Here's how the part is built. I have some questions about the finished solid (model axes, mm). Face numbers are marked on the shaded views. A direction names the side the tool comes from. Coordinates: 2 decimals unless noted, no trailing zeros. Write each loop counter-clockwise with the first axis right and the second up, starting at its lowest first coordinate (ties: lowest second). Pieces come first, ordered by that corner, then holes.
Item 1: I'm going to push flat-ended pins straight in: pin 1 Ø4 at (y, z) = (0, 8) entering from +X; pin 2 Ø4 at (y, z) = (14.5, 8.5) entering from +X; pin 3 Ø2.5 at (y, z) = (18, 7) entering from -X; pin 4 Ø1 at (x, z) = (5.5, 6.5) entering from -Y. Where does each tip first touch, or does it pass through?
Item 2: If we section it at C-C (y = -4): Please give me the cut outline in (x, z), then the cut area to 3 significant figures.
Item 3: For the marked faces 5, 6 and 7, which set-ups out of +Z, -Z, +X, -X, +Y, -Y let a thin tool reach every point of the face, with its end or its side?
Item 4: If we section it at B-B (z = 6): Please give me the cut outline in (x, y), then the cut area to 3 significant figures.
Item 5: If we section it at D-D (z = 8.25): Count the separate pieces of the cut face and the enclosed holes in it, then the cut area to 3 significant figures.
Item 6: We'd pull the mould along Y, two halves only. Please class the marked faces 1, 2, 3 and 4: +Y half, -Y half, draft (parallel to the pull), parting line (faces both ways), or undercut.
Item 7: If we section it at A-A (x = 0): Please give me the cut outline in (y, z), then the cut area to 3 significant figures.
Item 8: If I drill on line 1 (Y direction, x = 0, z = 2.75); line 2 (X direction, y = -6.5, z = 10.75); line 3 (Y direction, x = 0, z = 5.25), over which ranges is the centre line in solid material (lowest first)?
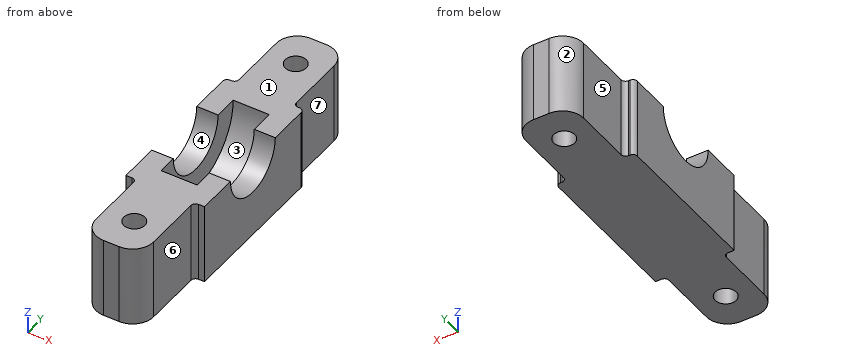
from build123d import *

# Parameters (mm, degrees)
F0_R     = 1.5
F0_W     = 5.1
F0_H     = 16.1
F1_DEPTH = 11.5
F3_DEPTH = 25


# Not quite as in the source:
# - a feature names something its author has since deleted; it is built from what else it names


with BuildPart() as f1:
    # F0 (on Top) → F1 (new body)
    with BuildSketch(Plane.XY):
        with BuildLine():
            ThreePointArc((5.5999997705, 10.465261464), (5.4140892248, 10.9140892248), (4.965261464, 11.0999997705))
            Line((4.965261464, 11.0999997705), (4.734738077, 11.0999997705))
            Line((4.734738077, 11.0999997705), (-4.734738077, 11.0999997705))
            Line((-4.734738077, 11.0999997705), (-4.965261464, 11.0999997705))
            ThreePointArc((-4.965261464, 11.0999997705), (-5.4140892248, 10.9140892248), (-5.5999997705, 10.465261464))
            Line((-5.5999997705, 10.465261464), (-5.5999997705, -10.465261464))
            ThreePointArc((-5.5999997705, -10.465261464), (-5.4140892248, -10.9140892248), (-4.965261464, -11.0999997705))
            Line((-4.965261464, -11.0999997705), (-4.734738077, -11.0999997705))
            Line((-4.734738077, -11.0999997705), (4.734738077, -11.0999997705))
            Line((4.734738077, -11.0999997705), (4.965261464, -11.0999997705))
            ThreePointArc((4.965261464, -11.0999997705), (5.4140892248, -10.9140892248), (5.5999997705, -10.465261464))
            Line((5.5999997705, -10.465261464), (5.5999997705, 10.465261464))
        make_face()
        Polygon((2.6, 8.1), (2.6, 0), (2.6, -8.1), (-2.6, -8.1), (-2.6, 8.1), align=None, mode=Mode.SUBTRACT)
        with BuildLine():
            Line((-4.734738077, 11.0999997705), (4.734738077, 11.0999997705))
            ThreePointArc((4.734738077, 11.0999997705), (4.2859103162, 11.2859103162), (4.0999997705, 11.734738077))
            Line((4.0999997705, 11.734738077), (4.0999997705, 20.0999997705))
            ThreePointArc((4.0999997705, 20.0999997705), (3.2213201141, 22.2213201141), (1.0999997705, 23.0999997705))
            Line((1.0999997705, 23.0999997705), (-1.0999997705, 23.0999997705))
            ThreePointArc((-1.0999997705, 23.0999997705), (-3.2213201141, 22.2213201141), (-4.0999997705, 20.0999997705))
            Line((-4.0999997705, 20.0999997705), (-4.0999997705, 11.734738077))
            ThreePointArc((-4.0999997705, 11.734738077), (-4.2859103162, 11.2859103162), (-4.734738077, 11.0999997705))
        make_face()
        with Locations((0, 18)):
            Circle(F0_R, mode=Mode.SUBTRACT)
        with BuildLine():
            ThreePointArc((4.0999997705, -11.734738077), (4.2859103162, -11.2859103162), (4.734738077, -11.0999997705))
            Line((4.734738077, -11.0999997705), (-4.734738077, -11.0999997705))
            ThreePointArc((-4.734738077, -11.0999997705), (-4.2859103162, -11.2859103162), (-4.0999997705, -11.734738077))
            Line((-4.0999997705, -11.734738077), (-4.0999997705, -20.0999997705))
            ThreePointArc((-4.0999997705, -20.0999997705), (-3.2213201141, -22.2213201141), (-1.0999997705, -23.0999997705))
            Line((-1.0999997705, -23.0999997705), (1.0999997705, -23.0999997705))
            ThreePointArc((1.0999997705, -23.0999997705), (3.2213201141, -22.2213201141), (4.0999997705, -20.0999997705))
            Line((4.0999997705, -20.0999997705), (4.0999997705, -11.734738077))
        make_face()
        with Locations((0, -18)):
            Circle(F0_R, mode=Mode.SUBTRACT)
        Polygon((2.6, -8.1), (2.6, 0), (2.6, 8.1), (-2.6, 8.1), (-2.6, -8.1), align=None)
        Rectangle(F0_W, F0_H, mode=Mode.SUBTRACT)
        Rectangle(F0_W, F0_H)
        with BuildLine():
            Line((5.5999997705, -11.0999997705), (5.5999997705, -10.465261464))
            ThreePointArc((5.5999997705, -10.465261464), (5.4140892248, -10.9140892248), (4.965261464, -11.0999997705))
            Line((4.965261464, -11.0999997705), (5.5999997705, -11.0999997705))
        make_face()
        with BuildLine():
            ThreePointArc((-4.965261464, -11.0999997705), (-5.4140892248, -10.9140892248), (-5.5999997705, -10.465261464))
            Line((-5.5999997705, -10.465261464), (-5.5999997705, -11.0999997705))
            Line((-5.5999997705, -11.0999997705), (-4.965261464, -11.0999997705))
        make_face()
    extrude(amount=F1_DEPTH)

    # F2 (on face) → F3 (cut)
    with BuildSketch(Plane.YZ.offset(5.5999997705)):
        with BuildLine():
            ThreePointArc((-5.3173691533, 11.5), (-0.3173691533, 6.5), (4.6826308467, 11.5))
            Line((4.6826308467, 11.5), (-5.3173691533, 11.5))
        make_face()
    extrude(amount=-F3_DEPTH, mode=Mode.SUBTRACT)

    # F4 (on face) → F5 (revolve, cut)
    with BuildSketch(Plane.XY.offset(11.5)):
        Polygon((2.55, 8.05), (-2.55, 8.05), (-2.55, 4.6826308467), (2.6, 4.6826308467), (2.6, 8.05), align=None)
        Polygon((2.6, 4.6826308467), (-2.55, 4.6826308467), (-2.55, 0), (0, 0), (2.6, 0), align=None)
    revolve(axis=Axis((0.025, 0, 11.5), (-1, 0, 0)), mode=Mode.SUBTRACT)


solid = f1.part
Answer list:
1. pin 1: stops at x = 5.6
1. pin 2: stops at x = 4.1
1. pin 3: stops at x = -4.1
1. pin 4: stops at y = -11.1
2. outline: (-5.6, 0) - (5.6, 0) - (5.6, 8.12) - (2.6, 8.12) - (2.6, 4.51) - (-2.55, 4.51) - (-2.55, 8.12) - (-5.6, 8.12) - close
2. area: 72.4 mm2
3. face 5: +Z, -Z, -X, +Y
3. face 6: +Z, -Z, +X, -Y
3. face 7: +Z, -Z, +X, +Y
4. outline: (-5.6, -11.1) - (-4.73, -11.1) arc R0.63 cw to (-4.1, -11.73) - (-4.1, -20.1) arc R3 ccw to (-1.1, -23.1) - (1.1, -23.1) arc R3 ccw to (4.1, -20.1) - (4.1, -11.73) arc R0.63 cw to (4.73, -11.1) - (5.6, -11.1) - (5.6, 10.47) arc R0.63 ccw to (4.97, 11.1) - (4.73, 11.1) arc R0.63 cw to (4.1, 11.73) - (4.1, 20.1) arc R3 ccw to (1.1, 23.1) - (-1.1, 23.1) arc R3 ccw to (-4.1, 20.1) - (-4.1, 11.73) arc R0.63 cw to (-4.73, 11.1) - (-4.97, 11.1) arc R0.63 ccw to (-5.6, 10.47) - close; hole (-2.55, -5.88) - (2.6, -5.88) - (2.6, 5.88) - (-2.55, 5.88) - close; hole circle Ø3 at (0, -18); hole circle Ø3 at (0, 18)
4. area: 363 mm2
5. separate pieces: 2
5. enclosed holes: 2
5. area: 302 mm2
6. face 1: draft
6. face 2: +Y half
6. face 3: undercut
6. face 4: undercut
7. outline: (-23.1, 0) - (-19.5, 0) - (-19.5, 11.5) - (-23.1, 11.5) - close; (-16.5, 0) - (16.5, 0) - (16.5, 11.5) - (8.05, 11.5) arc R8.05 cw to (-8.05, 11.5) - (-16.5, 11.5) - close; (19.5, 0) - (23.1, 0) - (23.1, 11.5) - (19.5, 11.5) - close
7. area: 361 mm2
8. line 1: y = -23.1 to -19.5, -16.5 to 16.5, 19.5 to 23.1
8. line 2: x = -5.6 to -2.55, 2.6 to 5.6
8. line 3: y = -23.1 to -19.5, -16.5 to -5.07, 5.07 to 16.5, 19.5 to 23.1
